For this review, take the finished solid that the model builds, in its own axes (mm). A direction names the side the tool comes from. Coordinates: 2 decimals unless noted, no trailing zeros. Write each loop counter-clockwise with the first axis right and the second up, starting at its lowest first coordinate (ties: lowest second). Pieces come first, ordered by that corner, then holes.
```python
from build123d import *

# Parameters (mm, degrees)
SKETCH3_R   = 32.4485
SKETCH3_R_2 = 26.2509
FILLET1_R   = 6.1976


with BuildPart() as part:
    # Sketch1 → Revolve1 (revolve)
    with BuildSketch(Plane.XY, mode=Mode.PRIVATE) as revolve1_sk:
        Polygon((-58.7375, -36.5125), (-54.6735, -32.4485), (-54.6735, -26.2509), (-58.7375, -30.0863), (-96.8375, -30.3149), (-96.8375, -36.5125), align=None)
    revolve(revolve1_sk.sketch.rotate(Axis((-96.8375, 0, 0), (1, 0, 0)), 270), axis=Axis((-96.8375, 0, 0), (1, 0, 0)))



with BuildPart() as body_2:
    # Sketch2 → Revolve2 (revolve)
    with BuildSketch(Plane.XY, mode=Mode.PRIVATE) as revolve2_sk:
        Polygon((30.3149, 96.8375), (30.0863, 58.7375), (26.2509, 54.6735), (32.4485, 54.6735), (36.5125, 58.7375), (36.5125, 96.8375), align=None)
    revolve(revolve2_sk.sketch.rotate(Axis((0, 0, 0), (0, 1, 0)), 90), axis=Axis((0, 0, 0), (0, 1, 0)))


with BuildPart() as part_1:
    add(part.part)

    add(body_2.part)  # Sweep1 merges body 2
    # Sweep1: sweep along a path in Sketch4
    with BuildLine(Plane.XY) as sweep1_path:
        ThreePointArc((-54.6735, 0), (-16.013497399, 16.013497399), (0, 54.6735))
    # Sketch3 → Sweep1 (sweep)
    with BuildSketch(Plane(origin=(-54.6735, 0, 0), x_dir=(0, 0, -1), z_dir=(1, 0, 0))):
        Circle(SKETCH3_R)
        Circle(SKETCH3_R_2, mode=Mode.SUBTRACT)
    sweep(path=sweep1_path.line)

    # Fillet1
    fillet1_edges = [part_1.edges().sort_by_distance(p)[0] for p in [
        (-54.6735, -32.4485, 0),
        (0, 54.6735, 32.4485),
        (0, 58.7375, 36.5125),
        (-58.7375, 0, -36.5125),
    ]]
    fillet(fillet1_edges, radius=FILLET1_R)


solid = part_1.part
```
Q1. Draft analysis for pull direction X (two halves, no side actions). For faces 4 (the flat face through (-96.838, -27.22, 13.69)), 5 (the conical face through (16.087, 54.871, 20.98)), 6 (the cylindrical face through (13.98, 79.32, -33.73)), state which applies: +X half, -X half, draft (parallel to the pull), parting line (faces both ways), or undercut.
Ans:
face 4: -X half
face 5: undercut
face 6: parting line
Q2. For probe 1 along Z at (x, y) = (13, 37); probe 2 along Y at (x, z) = (-55.5, -3.5); probe 3 along X at (y, z) = (69.5, -11), list the stretches that pass through material, from the lowest coordinate up.
Ans:
probe 1: z = -28.63 to -21.35, 21.35 to 28.63
probe 2: y = -33.26 to -26.8, 26.8 to 33.34
probe 3: x = -34.82 to -28.07, 28.07 to 34.82
Q3. Add section A-A (y = 85.5). State the section outline as (x, z) points (1 decimal), then the cut area to 3 significant figures.
Ans:
outline: circle Ø73 at (0, 0); hole circle Ø60.5 at (0, 0)
area: 1,310 mm2
Q4. Tool access review of faces 1 (the conical face through (29.48, 77.52, 6.55)), 2 (the conical face through (-56.58, -34.062, -4.472)), 3 (the conical face through (-78.05, 11.57, 27.9)): name each direction out of +Z, -Z, +X, -X, +Y, -Y from which nothing blocks a thin tool from reaching the whole face with its end or side.
Ans:
face 1: +Y
face 2: none
face 3: -X
Q5. Clearance check with flat-ended pins moving along their axes: pin 1 Ø1 at (x, z) = (-48, 5) entering from -Y; pin 2 Ø5 at (y, z) = (69.5, 4) entering from +X; pin 3 Ø3 at (x, y) = (-17, 16) entering from -Z. State where each tip first meets the part, or that it passes through.
Ans:
pin 1: stops at y = -31.89
pin 2: stops at x = 36.48
pin 3: stops at z = -32.45
Q6. Add section B-B (x = -70.5). State the section outline as (y, z) points (1 decimal), then the cut area to 3 significant figures.
Ans:
outline: circle Ø73 at (0, 0); hole circle Ø60.3 at (0, 0)
area: 1,330 mm2
